For this review, take the finished solid that the model builds, in its own axes (mm). Give positions to 0.01 mm unless a question says otherwise; leave off trailing zeros. Order: outer loops, then holes, each group sorted by start corner. A loop starts at its lowest first (then second) coordinate and runs counter-clockwise, first axis right, second up. Notation, with made-up numbers: (86, -17) -> (92, -17) arc R9 ccw to (92, -6) -> close; hole circle Ø10 at (-20.75, 58.25). An arc over 180 degrees is marked (long way). Return JSON: item names as keys, results as strings. Group by question number.
1) Add section C-C (y = 96). Give the boundary of the cut face in (x, z) (3 decimals).
2) Add section B-B (x = -13.75). Give the boundary of the cut face in (y, z) (3 decimals).
3) To check wall thickness, follow line 1 along X through (y, z) = (640, -7) (3 decimals); line 2 along Y through (x, z) = (-22.25, -23). State the ranges of each line that lie inside material, in increasing order.
4) Add section A-A (z = -13.5). Give the boundary of the cut face in (x, y) (3 decimals).
Autodesk Inventor part; units mm, degrees
ref_plane "YZ Plane" through (0, 0, 0) normal (1, 0, 0) x (0, 1, 0)
ref_plane "XZ Plane" through (0, 0, 0) normal (0, 1, 0) x (-1, 0, 0)
ref_plane "XY Plane" through (0, 0, 0) normal (0, 0, 1) x (1, 0, 0)
sketch "Sketch1" plane through (0, 0, 0) normal (0, 1, 0) x (-1, 0, 0)
  line L0 (0, 0) -> (25.4, 0)
  line L1 (25.4, 0) -> (25.4, -25.4)
  line L2 (25.4, -25.4) -> (0, -25.4)
  line L3 (0, -25.4) -> (0, 0)
  line L4 (3.175, -3.175) -> (22.225, -3.175)
  line L5 (22.225, -3.175) -> (22.225, -22.225)
  line L6 (22.225, -22.225) -> (3.175, -22.225)
  line L7 (3.175, -22.225) -> (3.175, -3.175)
  dimension "d0" = 25.4
  dimension "d1" = 25.4
  dimension "d2" = 3.175
extrude "Extrusion1" add sketch "Sketch1" along normal blind 762
chamfer "Chamfer1" distance 25.4 angle 45 2 edges at (-12.7, 762, 0) (-12.7, 0, 0)
properties part number "1x1x30"
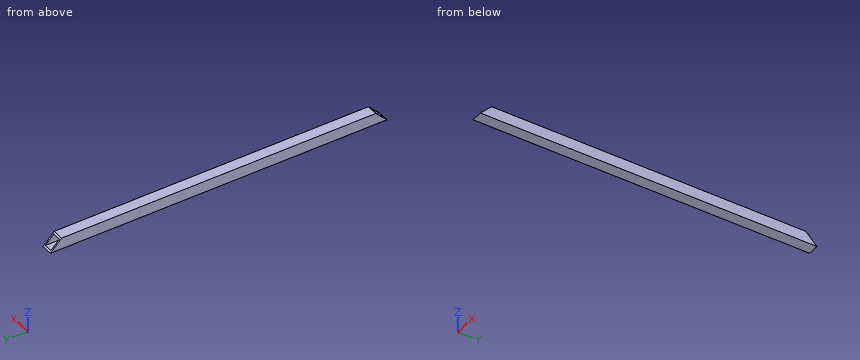
Evaluation:
{
 "1": {"outline": "(-25.4, -25.4) -> (0, -25.4) -> (0, 0) -> (-25.4, 0) -> close; hole (-22.225, -22.225) -> (-3.175, -22.225) -> (-3.175, -3.175) -> (-22.225, -3.175) -> close"},
 "2": {"outline": "(0, -25.4) -> (762, -25.4) -> (758.825, -22.225) -> (3.175, -22.225) -> close; (22.225, -3.175) -> (739.775, -3.175) -> (736.6, 0) -> (25.4, 0) -> close"},
 "3": {"line 1": "-25.4 to -22.225, -3.175 to 0", "line 2": "2.4 to 759.6"},
 "4": {"outline": "(-25.4, 11.9) -> (-22.225, 11.9) -> (-22.225, 750.1) -> (-25.4, 750.1) -> close; (-3.175, 11.9) -> (0, 11.9) -> (0, 750.1) -> (-3.175, 750.1) -> close"}
}
